Geometry: final body of the model. Coordinates: model frame, mm. Face numbers are marked on the shaded views. Coordinates: 2 decimals unless noted, no trailing zeros. Order: outer loops, then holes, each group sorted by start corner. A loop starts at its lowest first (then second) coordinate and runs counter-clockwise, first axis right, second up. Notation, with made-up numbers: (81.5, 9) -> (133.5, 9) arc R17 cw to (133.5, 41) -> close; hole circle Ø5 at (36.25, -13.5). An arc over 180 degrees is marked (long way). Answer in a Markdown table with one row per item. Add a question column.
1) Pull-direction query (Y, two-part tool) for the marked faces 1 and 2; classes: +Y half, -Y half, draft (parallel to the pull), parting line (faces both ways), or undercut.
2) Contact query for flat-ended pins moving along their axis: P1, Ø5.5, axis at x = -17.39, y = -10.62, coming from the +Z side; P2, Ø1, axis at x = 4, z = 1.5, coming from the +Y side; P3, Ø16, axis at x = 1.5, y = 7.5, coming from the +Z side; P4, Ø1.3, axis at x = 9.42, y = 9.65, coming from the +Z side. Output: stop coordinate, or through.
3) Section query A-A on y = 0. Return the cut outline in (x, z), then the cut area to 3 significant figures.
4) Ray query, line 1 (Y direction, x = 0, z = 5.6); line 2 (Z direction, x = 8, y = 3.5); line 3 (Y direction, x = 14, z = 5.5). Return the intervals inside material, ascending. Write a range as from..to.
5) Section query C-C on z = 1.75. Return the cut outline in (x, y).
```python
from build123d import *

# Parameters (mm, degrees)
F0_R      = 27.8603665739
F1_DEPTH  = 3.048
F4_R      = 26.2786257822
F5_DEPTH  = 1.016
F6_R      = 22.2176168744
F7_DEPTH  = 3.302
F9_R      = 15.773437446
F10_DEPTH = 2.032
F11_R     = 2.2956006308
F12_DEPTH = 21.336
F13_R     = 2.0464830212
F14_DEPTH = 25.4
F15_R     = 0.7900286513
F16_DEPTH = 25.4


# Not quite as in the source:
# - a fillet or chamfer that OpenCascade refuses, or shapes differently, is made with other operations: its cross-section is extruded or revolved along the edge and cut away or added


with BuildPart() as f1:
    # F0 (on Top) → F1 (new body)
    with BuildSketch(Plane.XY):
        Circle(F0_R)
    extrude(amount=F1_DEPTH)

    # F2: fillet of radius 5.08 on 1 edges, made by hand

    # F2_s1 → F2_t2 (revolve, cut)
    with BuildSketch(Plane.XZ):
        with BuildLine():
            ThreePointArc((27.8603665739, 0), (25.9869002599, 2.2182329348), (23.2044696678, 3.048))
            Line((23.2044696678, 3.048), (27.8603665739, 3.048))
            Line((27.8603665739, 3.048), (27.8603665739, 0))
        make_face()
    revolve(axis=Axis((0, 0, 3.048), (0, 0, 1)), mode=Mode.SUBTRACT)

    # F4 (on face) → F5 (join)
    with BuildSketch(Plane(origin=(0, 0, 0), x_dir=(1, 0, 0), z_dir=(0, 0, -1))):
        Circle(F4_R)
    extrude(amount=F5_DEPTH)

    # F6 (on face) → F7 (join)
    with BuildSketch(Plane.XY.offset(3.048)):
        Circle(F6_R)
    extrude(amount=F7_DEPTH)

    # F8: fillet of radius 5.08 on 1 edges, made by hand

    # F8_s1 → F8_t2 (revolve, cut)
    with BuildSketch(Plane.XZ):
        with BuildLine():
            ThreePointArc((22.2176168744, 3.048), (20.3549739793, 5.4436458882), (17.4589283996, 6.35))
            Line((17.4589283996, 6.35), (22.2176168744, 6.35))
            Line((22.2176168744, 6.35), (22.2176168744, 3.048))
        make_face()
    revolve(axis=Axis((0, 0, 6.35), (0, 0, 1)), mode=Mode.SUBTRACT)

    # F9 (on face) → F10 (cut)
    with BuildSketch(Plane.XY.offset(6.35)):
        Circle(F9_R)
    extrude(amount=-F10_DEPTH, mode=Mode.SUBTRACT)

    # F11 (on face) → F12 (cut)
    with BuildSketch(Plane.XY.offset(3.048)):
        with Locations((-17.1565320343, -10.5084851384)):
            Circle(F11_R)
    extrude(amount=-F12_DEPTH, mode=Mode.SUBTRACT)

    # F13 (on face) → F14 (cut)
    with BuildSketch(Plane.XY.offset(6.35)):
        with Locations((-17.3885338008, -10.6187639758)):
            Circle(F13_R)
    extrude(amount=-F14_DEPTH, mode=Mode.SUBTRACT)

    # F15 (on face) → F16 (cut)
    with BuildSketch(Plane.XY.offset(4.318)):
        with Locations((9.4199227169, 9.6543869004)):
            Circle(F15_R)
    extrude(amount=-F16_DEPTH, mode=Mode.SUBTRACT)


solid = f1.part
```
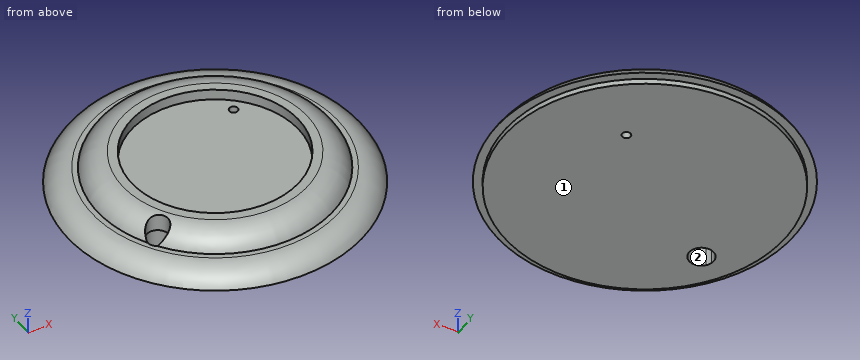
Result:
| question | item | result |
|---|---|---|
| 1 | face 1 | draft |
| 1 | face 2 | undercut |
| 2 | P1 | z = 6.35 |
| 2 | P2 | y = 26.99 |
| 2 | P3 | z = 4.32 |
| 2 | P4 | through |
| 3 | outline | (-27.86, 0) -> (-26.28, 0) -> (-26.28, -1.02) -> (26.28, -1.02) -> (26.28, 0) -> (27.86, 0) arc R5.08 ccw to (23.2, 3.05) -> (22.22, 3.05) arc R5.08 ccw to (17.46, 6.35) -> (15.77, 6.35) -> (15.77, 4.32) -> (-15.77, 4.32) -> (-15.77, 6.35) -> (-17.46, 6.35) arc R5.08 ccw to (-22.22, 3.05) -> (-23.2, 3.05) arc R5.08 ccw to start |
| 3 | area | 289 mm2 |
| 4 | line 1 | -20.12..-15.77, 15.77..20.12 |
| 4 | line 2 | -1.02..4.32 |
| 4 | line 3 | -14.66..-7.27, 7.27..14.66 |
| 5 | outline | circle Ø53.19 at (0, 0); hole (-19.4, -10.99) arc R2.05 ccw to (-18.95, -11.94) arc R2.3 ccw (long way) to start; hole circle Ø1.58 at (9.42, 9.65) |
